Design review of the part shown in the three views and the two pictorial views. Dimensions are in mm from the part's minimum x, y and z. Give positions to 0.01 mm unless a question says otherwise; leave off trailing zeros. Order: outer loops, then holes, each group sorted by start corner. A loop starts at its lowest first (then second) coordinate and runs counter-clockwise, first axis right, second up. Notation, with made-up numbers: (58, 43) -> (106, 43) arc R28 cw to (106, 74) -> close; hole circle Ø8 at (79.5, 61). An arc over 180 degrees is marked (long way). Use one line per item in the form item = value.
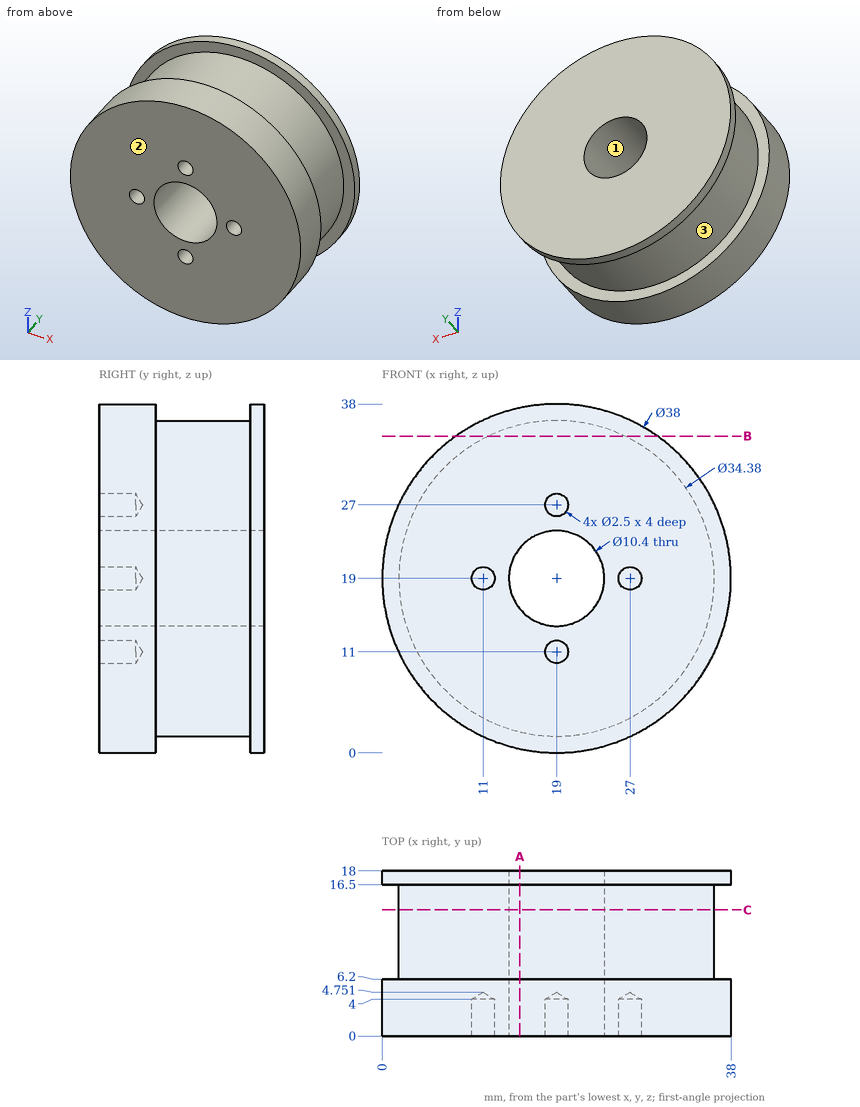
1. For pin 1 Ø1.5 at (y, z) = (13.5, 23) entering from -X; pin 2 Ø3 at (x, y) = (26, 10) entering from -Z; pin 3 Ø2 at (x, z) = (19, 11) entering from -Y, all flat-tipped, find the tip position at first contact; note any pin that passes through.
Values:
pin_1 = 2.12
pin_2 = 2.71
pin_3 = 4.15
2. Add section C-C on y = 13.75. Give the boundary of the cut face in (x, z).
Values:
outline = circle Ø34.38 at (19, 19); hole circle Ø10.4 at (19, 19)
3. For L1, parallel to X at y = 0.8, z = 19; L2, parallel to X at y = 6.25, z = 19; L3, parallel to Y at x = 29.5, z = 3.5, list the stretches that pass through material, from the lowest coordinate up.
Values:
L1 = 0 to 9.75, 12.25 to 13.8, 24.2 to 25.75, 28.25 to 38
L2 = 1.81 to 13.8, 24.2 to 36.19
L3 = 0 to 6.2, 16.5 to 18
4. Add section B-B on z = 34.5. Give the boundary of the cut face in (x, y).
Values:
outline = (8.01, 0) -> (29.99, 0) -> (29.99, 6.2) -> (26.43, 6.2) -> (26.43, 16.5) -> (29.99, 16.5) -> (29.99, 18) -> (8.01, 18) -> (8.01, 16.5) -> (11.57, 16.5) -> (11.57, 6.2) -> (8.01, 6.2) -> close
5. The part is to be moulded in two halves that separate along Z. For the marked faces 1, 2 and 3, say which applies: +Z half, -Z half, draft (parallel to the pull), parting line (faces both ways), or undercut.
Values:
face_1 = undercut
face_2 = draft
face_3 = parting line
6. Add section A-A on x = 15. Give the boundary of the cut face in (y, z).
Values:
outline = (0, 0.43) -> (6.2, 0.43) -> (6.2, 2.28) -> (16.5, 2.28) -> (16.5, 0.43) -> (18, 0.43) -> (18, 15.68) -> (0, 15.68) -> close; (0, 22.32) -> (18, 22.32) -> (18, 37.57) -> (16.5, 37.57) -> (16.5, 35.72) -> (6.2, 35.72) -> (6.2, 37.57) -> (0, 37.57) -> close
